Autodesk Inventor part; units mm, degrees
ref_plane "YZ Plane" through (0, 0, 0) normal (1, 0, 0) x (0, 1, 0)
ref_plane "XZ Plane" through (0, 0, 0) normal (0, 1, 0) x (-1, 0, 0)
ref_plane "XY Plane" through (0, 0, 0) normal (0, 0, 1) x (1, 0, 0)
sketch "Sketch1" plane through (0, 0, 0) normal (0, 0, 1) x (1, 0, 0)
  line L0 (0, 0) -> (76.2, 0)
  line L1 (76.2, 0) -> (76.2, 25.4)
  line L2 (76.2, 25.4) -> (0, 25.4)
  line L3 (0, 25.4) -> (0, 0)
  dimension "d0" = 76.2
  dimension "d1" = 25.4
extrude "Extrusion1" add sketch "Sketch1" along normal blind 14.2875
fillet "Fillet1" radius 2.54 8 edges at (38.1, 25.4, 14.2875) (38.1, 0, 14.2875) (76.2, 0, 7.1437) (76.2, 25.4, 7.1437) (0, 25.4, 7.1437) (0, 0, 7.1437) (38.1, 25.4, 0) (38.1, 0, 0)
sketch "Sketch2" plane through (0, 0, 14.2875) normal (0, 0, 1) x (1, 0, 0)
  line L0 (2.54, 2.54) -> (2.54, 22.86)
  line L1 (2.54, 12.7) -> (73.66, 12.7)
  line L2 (73.66, 22.86) -> (73.66, 2.54)
  circle A0 centre (38.1, 12.7) radius 3.175
  point P0 (0, 0)
  dimension "d5" = 6.35
extrude "Extrusion2" cut sketch "Sketch2" against normal blind 14.2875
thread "Thread1"
fillet "Fillet2" radius 7.1437 12 edges at (75.4561, 24.6561, 13.5436) (75.4561, 0.7439, 13.5436) (76.2, 12.7, 14.2875) (75.4561, 24.6561, 0.7439) (75.4561, 0.7439, 0.7439) (76.2, 12.7, 0) (0.7439, 0.7439, 13.5436) (0.7439, 24.6561, 13.5436) (0, 12.7, 14.2875) (0.7439, 0.7439, 0.7439) (0.7439, 24.6561, 0.7439) (0, 12.7, 0)
properties part number "bolt" material "Zinc"
Source: CAD feature listing. Evaluate the final solid. Frame: model axes, mm. Round coordinates to 2 decimals unless told otherwise and drop trailing zeros. Write each loop counter-clockwise with the first axis right and the second up, starting at its lowest first coordinate (ties: lowest second). Pieces come first, ordered by that corner, then holes. Notation, with made-up numbers: M 40,78.25 L 99,78.25 A28 cw 99,103.25 Z; hole C 52.25,-14.75 d2. An arc over 180 degrees is marked long. Use CSV: the item, a comma, the result in double quotes. Start each with the question number.
Q1. Cut plane A-A on x = 38.1. Output: boundary loops of the cut face in (y, z) (1 decimal).
Q2. Cut plane D-D on x = 48. Output: boundary loops of the cut face in (y, z).
Q3. First-contact query: P1, Ø1.5, axis at y = 5.5, z = 5, coming from the +X side; P2, Ø8, axis at y = 14.5, z = 11.5, coming from the +X side; P3, Ø5.5, axis at x = 38.1, y = 12.7, coming from the +Z side. Flat tips, straight axial feed; report the tip coordinate or a pass-through.
Q4. Line query: line 1 (Y direction, x = 38.1, z = 8.5) (3 decimals); line 2 (X direction, y = 12.7, z = 8.25) (3 decimals); line 3 (Y direction, x = 36, z = 1.25). Output: solid intervals per line, ascending. Write a range as from..to.
Results found:
1,outline,"M 0,2.5 A2.5 ccw 2.5,0 L 9.5,0 L 9.5,14.3 L 2.5,14.3 A2.5 ccw 0,11.7 Z; M 15.9,0 L 22.9,0 A2.5 ccw 25.4,2.5 L 25.4,11.7 A2.5 ccw 22.9,14.3 L 15.9,14.3 Z"
2,outline,"M 0,2.54 A2.54 ccw 2.54,0 L 22.86,0 A2.54 ccw 25.4,2.54 L 25.4,11.75 A2.54 ccw 22.86,14.29 L 2.54,14.29 A2.54 ccw 0,11.75 Z"
3,P1,"x = 76.06"
3,P2,"x = 76.19"
3,P3,"through"
4,line 1,"0..9.525, 15.875..25.4"
4,line 2,"0.086..34.925, 41.275..76.114"
4,line 3,"0.35..10.32, 15.08..25.05"
